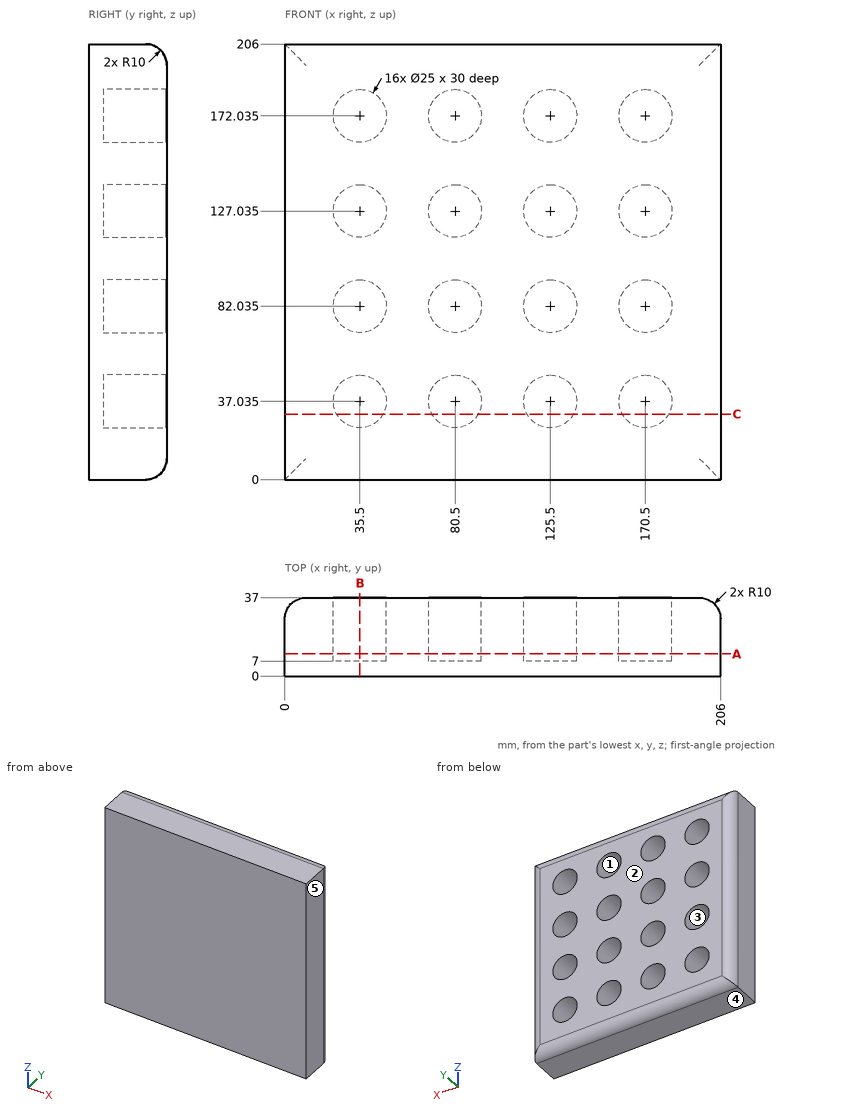
Can you work these out from the drawing? Everything is in mm from the part's minimum corner. A direction names the side the tool comes from. Coordinates: 2 decimals unless noted, no trailing zeros. Loops run counter-clockwise (first coordinate to the right, second up) from the corner with the lowest first, then second, coordinate; pieces in that order, holes last. Notation, with made-up numbers: (-9.5, -22.75) - (22.5, -22.75) arc R29 ccw to (22.5, 11.25) - close; hole circle Ø10 at (32, 0.5). An arc over 180 degrees is marked (long way). Use a Markdown table: item, result.
Item 1: We'd pull the mould along X, two halves only. Please class the marked faces 3, 4 and 5: released by +X, released by -X, zero draft, split by the parting line, or undercut.
Numbers:
| item | result |
|---|---|
| face 3 | undercut |
| face 4 | zero draft |
| face 5 | released by +X |
Item 2: I want a section at A-A on y = 10.5. Give the number of separate pieces and of enclosed holes in the cut face, and give its area (3 significant figures).
Numbers:
| item | result |
|---|---|
| separate pieces | 1 |
| enclosed holes | 16 |
| area | 34,600 mm2 |
Item 3: For the marked faces 1 and 2, which set-ups out of +Z, -Z, +X, -X, +Y, -Y let a thin tool reach every point of the face, with its end or its side?
Numbers:
| item | result |
|---|---|
| face 1 | +Y |
| face 2 | +Z, -Z, +X, -X, +Y |
Item 4: I want a section at B-B on x = 35.5. Please give me the cut outline in (y, z) (1 decimal).
Numbers:
| item | result |
|---|---|
| outline | (0, 0) - (27, 0) arc R10 ccw to (37, 10) - (37, 24.5) - (7, 24.5) - (7, 49.5) - (37, 49.5) - (37, 69.5) - (7, 69.5) - (7, 94.5) - (37, 94.5) - (37, 114.5) - (7, 114.5) - (7, 139.5) - (37, 139.5) - (37, 159.5) - (7, 159.5) - (7, 184.5) - (37, 184.5) - (37, 196) arc R10 ccw to (27, 206) - (0, 206) - close |
Item 5: Will these pins go through, and if not, where does the flat tip stop? pin 1 (15 mm diameter, centred on x = 170.5, z = 82.03, fed in from +Y); pin 2 (8 mm diameter, centred on y = 32, z = 171, fed in from -X).
Numbers:
| item | result |
|---|---|
| pin 1 | stops at y = 7 |
| pin 2 | stops at x = 0.05 |
Item 6: If I drill on probe 1 along Z at (x, y) = (170, 18) (1 decimal); probe 2 along Z at (x, y) = (136.5, 9.5); probe 3 along X at (y, z) = (30, 161.5), over which ranges is the centre line in solid material (lowest first)? Write a range as from..to.
Numbers:
| item | result |
|---|---|
| probe 1 | z = 0..24.5, 49.5..69.5, 94.5..114.5, 139.5..159.5, 184.5..206 |
| probe 2 | z = 0..31.1, 42.97..76.1, 87.97..121.1, 132.97..166.1, 177.97..206 |
| probe 3 | x = 0.46..28.77, 42.23..73.77, 87.23..118.77, 132.23..163.77, 177.23..205.54 |
Item 7: I want a section at C-C on z = 31. Please give me the cut outline in (x, y).
Numbers:
| item | result |
|---|---|
| outline | (0, 0) - (206, 0) - (206, 27) arc R10 ccw to (196, 37) - (181.45, 37) - (181.45, 7) - (159.55, 7) - (159.55, 37) - (136.45, 37) - (136.45, 7) - (114.55, 7) - (114.55, 37) - (91.45, 37) - (91.45, 7) - (69.55, 7) - (69.55, 37) - (46.45, 37) - (46.45, 7) - (24.55, 7) - (24.55, 37) - (10, 37) arc R10 ccw to (0, 27) - close |
